The model under review builds one solid part; all positions refer to its coordinate system, in mm. Coordinates: 2 decimals unless noted, no trailing zeros. Order: outer loops, then holes, each group sorted by start corner. A loop starts at its lowest first (then second) coordinate and runs counter-clockwise, first axis right, second up. Notation, with made-up numbers: M -26.75,69 L 24.25,69 A11 ccw 24.25,77 Z; hole C 25,-36.75 d3. An arc over 180 degrees is marked long. Write each question's results on one line, items separated by ' | '.
from build123d import *

# Parameters (mm, degrees)
F2_R     = 2.54
F3_R     = 2.159
F4_DEPTH = 127


# Not quite as in the source:
# - a fillet or chamfer that OpenCascade refuses, or shapes differently, is made with other operations: its cross-section is extruded or revolved along the edge and cut away or added


with BuildPart() as f1:
    # F0 (on Top) → F1 (revolve)
    with BuildSketch(Plane.XY):
        with BuildLine():
            Line((0, 2.794), (0, 0))
            Line((0, 0), (139.7, 0))
            Line((139.7, 0), (139.7, 6.35))
            Line((139.7, 6.35), (31.75, 6.35))
            ThreePointArc((31.75, 6.35), (21.3842908829, 5.6416689079), (11.0185817658, 6.35))
            ThreePointArc((11.0185817658, 6.35), (10.9918000406, 5.5558048596), (11.0379582651, 4.7625))
            Line((11.0379582651, 4.7625), (0, 2.794))
        make_face()
    revolve(axis=Axis((69.85, 0, 0), (1, 0, 0)))

    # F2
    f2_edges = [f1.edges().sort_by_distance(p)[0] for p in [
        (139.7, -6.35, 0),
    ]]
    fillet(f2_edges, radius=F2_R)

    # F3 (on face) → F4 (cut)
    with BuildSketch(Plane(origin=(0, 0, 0), x_dir=(0, -1, 0), z_dir=(-1, 0, 0))):
        Circle(F3_R)
    extrude(amount=-F4_DEPTH, mode=Mode.SUBTRACT)

    # F5: fillet of radius 3.175 on 1 edges, made by hand

    # F5_s1 → F5_t2 (revolve, cut)
    with BuildSketch(Plane.XY):
        with BuildLine():
            ThreePointArc((13.886159803, 6.0114768317), (12.2986630958, 5.7596010622), (11.0379582651, 4.7625))
            Line((11.0379582651, 4.7625), (10.9872426769, 4.8007122901))
            ThreePointArc((10.9872426769, 4.8007122901), (10.9283047702, 5.5550298573), (10.9552829498, 6.3550507327))
            Line((10.9552829498, 6.3550507327), (11.0272198567, 6.4129097241))
            ThreePointArc((11.0272198567, 6.4129097241), (12.4582117618, 6.2302164435), (13.8924082455, 6.0746686585))
            Line((13.8924082455, 6.0746686585), (13.886159803, 6.0114768317))
        make_face()
    revolve(axis=Axis((11.0185817658, 0, 0), (1, 0, 0)), mode=Mode.SUBTRACT)


solid = f1.part
1) Take a section at A-A on x = 52.5. State the section outline as (y, z) points.
Solutions:
outline: C 0,0 d12.7; hole C 0,0 d4.32
2) Take a section at B-B on x = 23. State the section outline as (y, z) points.
Solutions:
outline: C 0,0 d11.32; hole C 0,0 d4.32
3) For pin 1 (4 mm diameter, centred on x = 41.5, z = -4, fed in from +Y); pin 2 (4 mm diameter, centred on x = 23, y = -3.5, fed in from -Z); pin 3 (5 mm diameter, centred on x = 108.5, z = -3.5, fed in from -Y), all flat-tipped, find the tip position at first contact; note any pin that passes through.
Solutions:
pin 1: y = 6.03 | pin 2: z = -5.46 | pin 3: y = -6.27
4) The part is to be moulded in two halves that separate along Z. For faces 1 (the conical face through (4.22, 3.38, 1.07)), 2 (the flat face through (139.7, 0, 0)), 3 (the flat face through (127, 0, 0)), 4 (the cylindrical face through (62.61, 0.28, 2.14)), say which applies: pulls with the +Z half, pulls with the -Z half, needs draft (parallel to the pull), parting line crosses it, or undercut.
Solutions:
face 1: parting line crosses it | face 2: needs draft | face 3: undercut | face 4: undercut
5) To check wall thickness, follow line 1 along Z through (x, y) = (90.5, 0); line 2 along Y through (x, z) = (64.5, -0.25); line 3 along Y through (x, z) = (8, -0.25). State the ranges of each line that lie inside material, in increasing order.
Solutions:
line 1: -6.35 to -2.16, 2.16 to 6.35 | line 2: -6.35 to -2.14, 2.14 to 6.35 | line 3: -4.21 to -2.14, 2.14 to 4.21
